from build123d import *

# Parameters (mm, degrees)
ESQUISSE2_R                  = 1.5
ENL_V_MAT_EXTRU_1_DEPTH      = 89.606546076
R_P_TITION_CIRCULAIRE1_COUNT = 4
ESQUISSE6_R                  = 1.5
ENL_V_MAT_EXTRU_5_DEPTH      = 3
R_P_TITION_CIRCULAIRE4_COUNT = 3


with BuildPart() as part:
    # Esquisse1 → Base-Révolution (revolve)
    with BuildSketch(Plane(origin=(0, 0, 0), x_dir=(0, 0, -1), z_dir=(1, 0, 0)), mode=Mode.PRIVATE) as base_r_volution_sk:
        with BuildLine():
            Line((0, 56.6), (-22.05, 56.6))
            ThreePointArc((-22.05, 56.6), (-38, 40.65), (-22.05, 24.7))
            Line((-22.05, 24.7), (-22.05, 25.3))
            ThreePointArc((-22.05, 25.3), (-37.4, 40.65), (-22.05, 56))
            Line((-22.05, 56), (0, 56))
            Line((0, 56), (0, 56.6))
        make_face()
    revolve(base_r_volution_sk.sketch.rotate(Axis((0, 0, 53.003727506), (0, 0, -1)), 90), axis=Axis((0, 0, 53.003727506), (0, 0, -1)))

    # Esquisse2 → Enlèv. mat.-Extru.1 (cut, through all)
    with BuildSketch(Plane(origin=(0, 0, 0), x_dir=(1, 0, 0), z_dir=(0, 1, 0))):
        with Locations(Location((0, -2.5, 0), (0, 0, 270))):
            Circle(ESQUISSE2_R)
    enl_v_mat_extru_1 = extrude(amount=-ENL_V_MAT_EXTRU_1_DEPTH, mode=Mode.SUBTRACT)

    # Répétition circulaire1: Enlèv. mat.-Extru.1 ×4 about axis
    r_p_tition_circulaire1_axis = Axis((0, 0, 53.003727506), (0, 0, -1))
    for i in range(1, R_P_TITION_CIRCULAIRE1_COUNT):
        add(enl_v_mat_extru_1.rotate(r_p_tition_circulaire1_axis, i * 360 / R_P_TITION_CIRCULAIRE1_COUNT), mode=Mode.SUBTRACT)

    # Esquisse6 → Enlèv. mat.-Extru.5 (cut)
    with BuildSketch(Plane(origin=(0, -7.41473671, 12.842700706), x_dir=(-1, 0, 0), z_dir=(0, 0.49999999999999806, -0.8660254037844397))):
        with Locations(Location((0, 45.356406461, 0), (0, 0, 292.170563159))):
            Circle(ESQUISSE6_R)
    enl_v_mat_extru_5 = extrude(amount=ENL_V_MAT_EXTRU_5_DEPTH, mode=Mode.SUBTRACT)

    # Répétition circulaire4: Enlèv. mat.-Extru.5 ×3 about axis
    r_p_tition_circulaire4_axis = Axis((0, 0, 53.003727506), (0, 0, -1))
    for i in range(1, R_P_TITION_CIRCULAIRE4_COUNT):
        add(enl_v_mat_extru_5.rotate(r_p_tition_circulaire4_axis, i * 360 / R_P_TITION_CIRCULAIRE4_COUNT), mode=Mode.SUBTRACT)


solid = part.part
CAD build for the part. Positions are in the model's coordinates, mm. A direction names the side the tool comes from. Round coordinates to 2 decimals unless told otherwise and drop trailing zeros. Write each loop counter-clockwise with the first axis right and the second up, starting at its lowest first coordinate (ties: lowest second). Pieces come first, ordered by that corner, then holes. Notation, with made-up numbers: M -36.5,-24 L -16.5,-24 A26 cw -16.5,-9 Z; hole C 56,57.25 d1. An arc over 180 degrees is marked long. Put each result on its own line as item: value. Start each with the question number.
1) Drill centre lines: probe 1 along Y at (x, z) = (0, 12); probe 2 along X at (y, z) = (-8, 35); probe 3 along Y at (x, z) = (-50, 21.5). Where is each one in solid material? Low to high. Write a range as [from, to].
2) Pull direction Y, two halves, no side cores. Call faces 3 (the cylindrical face through (56.29, 0.07, 1)), 4 (the cylindrical face through (0.07, -56.29, 1)), 5 (the cylindrical face through (26.117, 50.214, 11.179)): pulls with the +Y half, pulls with the -Y half, needs draft (parallel to the pull), parting line crosses it, or undercut.
3) Pin check, flat tips, straight feed: pin 1 Ø1 at (x, z) = (-30.5, 26.5) entering from +Y; pin 2 Ø1 at (y, z) = (31, 33.5) entering from -X; pin 3 Ø8 at (y, z) = (-14.5, 22) entering from +X; pin 4 Ø3.5 at (y, z) = (0, 2.5) entering from -X. Stop position of each tip, or through.
4) Saw through at C-C, the plane z = 29. Write the cut outline in (x, y), and give its area (3 significant figures).
5) Saw through at A-A, the plane y = 0. Write the cut outline in (x, z), and give its area (3 significant figures).
6) Saw through at D-D, the plane z = 15.5. Write the cut outline in (x, y), and give its area (3 significant figures).
7) 3-axis set-ups, long thin cutter, end or side, ignore diameter. For faces 1 (the cylindrical face through (28.615, -17.103, 35.804)), 2 (the cylindrical face through (25.84, 49.68, 10.87)): which of +Z, -Z, +X, -X, +Y, -Y reach the whole face in a straight line?
8) Saw through at B-B, the plane z = 2.5. Write the cut outline in (x, y), and give its area (3 significant figures).
Resolved:
1. probe 1: [-56.6, -56], [56, 56.6]
1. probe 2: [-49.32, -48.23], [-31.41, -30.3], [30.3, 31.41], [48.23, 49.32]
1. probe 3: [-26.52, -25.22], [25.22, 26.52]
2. face 3: undercut
2. face 4: needs draft
2. face 5: parting line crosses it
3. pin 1: y = 47.29
3. pin 2: x = -42.16
3. pin 3: x = 55.62
3. pin 4: x = -56.6
4. outline: C 0,0 d110.01; C 0,0 d53.93; hole C 0,0 d108.67; hole C 0,0 d52.59
4. area: 342 mm²
5. outline: M -56.6,0 L -56,0 L -56,1 L -56.6,1 Z; M -56.6,4 L -56,4 L -56,22.05 A15.35 cw -25.3,22.05 L -24.7,22.05 A15.95 ccw -56.6,22.05 Z; M 24.7,22.05 L 25.3,22.05 A15.35 cw 56,22.05 L 56,4 L 56.6,4 L 56.6,22.05 A15.95 ccw Z; M 56,0 L 56.6,0 L 56.6,1 L 56,1 Z
5. area: 81.9 mm²
6. outline: C 0,0 d113.2; hole C 0,0 d112
6. area: 212 mm²
7. face 1: none
7. face 2: -Z
8. outline: M -56.58,-1.5 A56.6 ccw -1.5,-56.58 L -1.5,-55.98 A56 cw -55.98,-1.5 Z; M -56.58,1.5 L -55.98,1.5 A56 cw -1.5,55.98 L -1.5,56.58 A56.6 ccw Z; M 1.5,-56.58 A56.6 ccw 56.58,-1.5 L 55.98,-1.5 A56 cw 1.5,-55.98 Z; M 1.5,55.98 A56 cw 55.98,1.5 L 56.58,1.5 A56.6 ccw 1.5,56.58 Z
8. area: 205 mm²
